Source: CAD feature listing. Evaluate the final solid. Frame: model axes, mm. Face numbers are marked on the shaded views. Round coordinates to 2 decimals unless told otherwise and drop trailing zeros. Order: outer loops, then holes, each group sorted by start corner. A loop starts at its lowest first (then second) coordinate and runs counter-clockwise, first axis right, second up. Notation, with made-up numbers: (39.25, -32.5) - (92.25, -32.5) arc R25 cw to (92.25, 3.5) - close; hole circle Ø4 at (36.25, -31.5). An arc over 180 degrees is marked (long way). Put each result on its own line as item: value. Start each with the question number.
1) Line query: probe 1 along X at (y, z) = (10, 0.5); probe 2 along X at (y, z) = (10, 3.05); probe 3 along Y at (x, z) = (25, 3.35). Output: solid intervals per line, ascending. Write a range as [from, to].
2) Section D-D on z = 2.95. Output: boundary loops of the cut face in (x, y).
3) Section C-C on y = 6. Output: boundary loops of the cut face in (x, z), then the cut area to 3 significant figures.
4) Section A-A on x = 10.5. Output: boundary loops of the cut face in (y, z).
5) Section B-B on y = 10. Output: boundary loops of the cut face in (x, z).
6) Mould query, pull axis Y, two halves, no side actions, for the marked faces 1, 2 and 3. Classes: +Y half, -Y half, draft (parallel to the pull), parting line (faces both ways), or undercut.
Autodesk Inventor part; units mm, degrees
ref_plane "YZ Plane" through (0, 0, 0) normal (1, 0, 0) x (0, 1, 0)
ref_plane "XZ Plane" through (0, 0, 0) normal (0, 1, 0) x (-1, 0, 0)
ref_plane "XY Plane" through (0, 0, 0) normal (0, 0, 1) x (1, 0, 0)
sketch "Sketch1" plane through (0, 0, 0) normal (0, 0, 1) x (1, 0, 0)
  line L0 (0, 0) -> (50, 0)
  line L1 (50, 0) -> (50, 20)
  line L2 (50, 20) -> (0, 20)
  line L3 (0, 20) -> (0, 0)
  dimension "d0" = 50
  dimension "d1" = 20
extrude "Extrusion1" add sketch "Sketch1" along normal blind 4
sketch "Sketch2" plane through (0, 0, 4) normal (0, 0, 1) x (1, 0, 0)
  line L0 (50, 20) -> (0, 20)
  line L1 (0, 20) -> (0, 0)
  point P0 (25, 10)
  dimension "d11" = 10
  dimension "d12" = 25
hole "Hole1" at (25, 10, 4) direction (0, 0, -1) diameter 11 depth 4 tip angle 118 counterbore diameter 16.4 counterbore depth 2
sketch "Sketch3" plane through (0, 0, 4) normal (0, 0, 1) x (1, 0, 0)
  line L0 (50, 0) -> (50, 20)
  line L1 (50, 20) -> (0, 20)
  point P0 (0, 0)
  point P1 (39.5, 10)
  dimension "d21" = 10.5
  dimension "d22" = 10
hole "Hole2" at (39.5, 10, 4) direction (0, 0, -1) diameter 4 end through all
sketch "Sketch4" plane through (0, 0, 4) normal (0, 0, 1) x (1, 0, 0)
  line L0 (0, 0) -> (50, 0)
  line L1 (50, 0) -> (50, 20)
  point P0 (39.5, 5.9723)
  dimension "d30" = 5.9723
  dimension "d31" = 10.5
hole "Hole3" at (39.5, 5.9723, 4) direction (0, 0, -1) diameter 4 end through all
sketch "Sketch5" plane through (0, 0, 4) normal (0, 0, 1) x (1, 0, 0)
  line L0 (50, 20) -> (0, 20)
  line L1 (0, 20) -> (0, 0)
  point P0 (10.5, 10)
  dimension "d46" = 10
  dimension "d47" = 10.5
hole "Hole4" at (10.5, 10, 4) direction (0, 0, -1) diameter 4 end through all
sketch "Sketch6" plane through (0, 0, 4) normal (0, 0, 1) x (1, 0, 0)
  line L0 (0, 20) -> (0, 0)
  line L1 (0, 0) -> (50, 0)
  point P0 (10.5, 5.9723)
  dimension "d48" = 10.5
  dimension "d49" = 5.9723
hole "Hole5" at (10.5, 5.9723, 4) direction (0, 0, -1) diameter 4 end through all
delete faces "Delete Face1" heal yes whole lump no faces at (10.8208, 3.9982, 2.6667)
delete faces "Delete Face2" heal yes whole lump no faces at (40.1333, 4.0752, 2.6667)
properties part number "bottom"
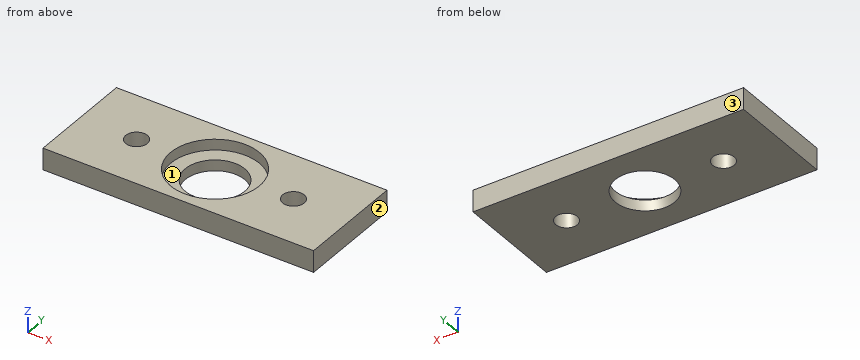
Answer sheet:
1. probe 1: [0, 8.5], [12.5, 19.5], [30.5, 37.5], [41.5, 50]
1. probe 2: [0, 8.5], [12.5, 16.8], [33.2, 37.5], [41.5, 50]
1. probe 3: [0, 1.8], [18.2, 20]
2. outline: (0, 0) - (50, 0) - (50, 20) - (0, 20) - close; hole circle Ø4 at (10.5, 10); hole circle Ø16.4 at (25, 10); hole circle Ø4 at (39.5, 10)
3. outline: (0, 0) - (21.23, 0) - (21.23, 2) - (17.84, 2) - (17.84, 4) - (0, 4) - close; (28.77, 0) - (50, 0) - (50, 4) - (32.16, 4) - (32.16, 2) - (28.77, 2) - close
3. area: 156 mm^2
4. outline: (0, 0) - (8, 0) - (8, 4) - (0, 4) - close; (12, 0) - (20, 0) - (20, 4) - (12, 4) - close
5. outline: (0, 0) - (8.5, 0) - (8.5, 4) - (0, 4) - close; (12.5, 0) - (19.5, 0) - (19.5, 2) - (16.8, 2) - (16.8, 4) - (12.5, 4) - close; (30.5, 0) - (37.5, 0) - (37.5, 4) - (33.2, 4) - (33.2, 2) - (30.5, 2) - close; (41.5, 0) - (50, 0) - (50, 4) - (41.5, 4) - close
6. face 1: undercut
6. face 2: draft
6. face 3: +Y half
